Autodesk Inventor part; units mm, degrees
ref_plane "Work Plane1" through (0, 2, 0) normal (0, 1, 0) x (1, 0, 0)
ref_plane "YZ Plane" through (0, 0, 0) normal (1, 0, 0) x (0, 1, 0)
ref_plane "XZ Plane" through (0, 0, 0) normal (0, 1, 0) x (-1, 0, 0)
sketch "Sketch1" plane through (0, 0, 0) normal (0, 1, 0) x (-1, 0, 0)
  line L0 (60, 60) -> (-60, 60)
  line L1 (-60, 60) -> (-60, -60)
  line L2 (-60, -60) -> (60, -60)
  line L3 (60, -60) -> (60, 60)
  line L4 (60, 60) -> (-60, -60) construction
  line L5 (-60, 60) -> (60, -60) construction
  point P0 (0, 0)
  dimension "d0" = 120
  dimension "d1" = 120
extrude "Extrusion1" add sketch "Sketch1" along normal blind 2
ref_plane "Work Plane1" through (0, 2, 0) normal (0, 1, 0) x (1, 0, 0)
sketch "Sketch2" plane through (0, 2, 0) normal (0, 1, 0) x (1, 0, 0)
  line L0 (60, 60) -> (-60, 60)
  line L1 (59.4693, -59.8704) -> (-60, 60)
  circle A0 centre (-50, 50) radius 2
  line L2 (0, 60) -> (0, 51.4464)
  circle A1 centre (50, 50) radius 2
  line L3 (60, -60) -> (60, 60)
  line L4 (60, 0) -> (52.6499, 0)
  circle A2 centre (50, -50) radius 2
  line L5 (-60, 60) -> (-60, -60)
  line L6 (-60, 0) -> (-53.051, 0)
  circle A3 centre (-50, -50) radius 2
  point P0 (0, 0)
  dimension "d5" = 4
extrude "Extrusion2" cut sketch "Sketch2" against normal through all
thread "Thread1"
properties part number "PCB"
Design review of the part built by this model. Coordinates are the model's own, in mm. Round coordinates to 2 decimals unless told otherwise and drop trailing zeros. Write each loop counter-clockwise with the first axis right and the second up, starting at its lowest first coordinate (ties: lowest second). Pieces come first, ordered by that corner, then holes. Notation, with made-up numbers: (49, 82) - (105, 82) arc R22 ccw to (105, 92) - close; hole circle Ø7 at (-34.5, -15). An arc over 180 degrees is marked (long way). Return JSON: item names as keys, results as strings. Group by question number.
Item 1: Insertion check: P1, Ø3, axis at x = -50, z = -50, coming from the +Y side. The pin has a flat end and moves straight along its axis. Give the tip position at first contact, or say it passes through.
Item 2: We need section B-B on z = -50. Write out the cut boundary in (x, y), and give its area (3 significant figures).
Item 3: The part is to be moulded in two halves that separate along X. For faces 1 (the face through (1, 0, 1)), 2 (the face through (50.923, 1.014, -48.226)), 3 (the face through (50.923, 1.014, 51.774)), say which applies: pulls with the +X half, pulls with the -X half, needs draft (parallel to the pull), parting line crosses it, or undercut.
Item 4: For probe 1 along X at (y, z) = (0.4, -50); probe 2 along Z at (x, y) = (50.5, 0.7), list the stretches that pass through material, from the lowest coordinate up. Write a range as [from, to].
Item 5: We need section A-A on x = 50. Write out the cut boundary in (y, z).
Model answer:
{
 "1": {"P1": "passes through"},
 "2": {"outline": "(-60, 0) - (-52, 0) - (-52, 2) - (-60, 2) - close; (-48, 0) - (48, 0) - (48, 2) - (-48, 2) - close; (52, 0) - (60, 0) - (60, 2) - (52, 2) - close", "area": "224 mm²"},
 "3": {"face 1": "needs draft", "face 2": "undercut", "face 3": "undercut"},
 "4": {"probe 1": "x = [-60, -52], [-48, 48], [52, 60]", "probe 2": "z = [-60, -51.94], [-48.06, 48.06], [51.94, 60]"},
 "5": {"outline": "(0, -60) - (2, -60) - (2, -52) - (0, -52) - close; (0, -48) - (2, -48) - (2, 48) - (0, 48) - close; (0, 52) - (2, 52) - (2, 60) - (0, 60) - close"}
}
